from build123d import *

# Parameters (mm, degrees)
F1_DEPTH = 1.5
F2_DEPTH = 5
F3_ANGLE = 120
F4_ANGLE = 120
F6_DEPTH = 3


with BuildPart() as f1:
    # F0 (on Top) → F1 (new body)
    with BuildSketch(Plane.XY):
        Polygon((4.7835907286, 2.7618073949), (16.4544826719, 9.5), (9.3638996784, 13.59375), (8.2350135643, 12.5134618943), (6.7194691076, 13.3884618943), (7.0905829935, 14.90625), (0, 19), (0, 5.5236147897), (1.5310889132, 4.6396401935), (1.5310889132, 14.6519237886), (11.9233937587, 8.6519237886), (3.2525018154, 3.6457819911), align=None)
        Polygon((0, 0), (4.7835907286, 2.7618073949), (3.2525018154, 3.6457819911), (1.5310889132, 2.6519237886), (1.5310889132, 4.6396401935), (0, 5.5236147897), align=None)
        Polygon((-4.7835907286, 2.7618073949), (0, 0), (0, 5.5236147897), (-1.5310889132, 4.6396401935), (-1.5310889132, 2.6519237886), (-3.2525018154, 3.6457819911), align=None)
        Polygon((-1.5310889132, 4.6396401935), (0, 5.5236147897), (0, 19), (-6.7116968793, 15.125), (-7.0364564057, 14.9375), (-5.8534437039, 13.8884618943), (-9.101038968, 12.0134618943), (-9.4180262662, 13.5625), (-9.7427857926, 13.375), (-16.4544826719, 9.5), (-4.7835907286, 2.7618073949), (-3.2525018154, 3.6457819911), (-11.9233937587, 8.6519237886), (-1.5310889132, 14.6519237886), align=None)
    extrude(amount=F1_DEPTH)

    # F0 (on Top) → F2 (join)
    with BuildSketch(Plane.XY):
        Polygon((8.2350135643, 12.5134618943), (9.3638996784, 13.59375), (9.0888552775, 13.7525469589), (8.1894266762, 12.8918383296), (7.0699461568, 13.5381707088), (7.3656273944, 14.7474530411), (7.0905829935, 14.90625), (6.7194691076, 13.3884618943), align=None)
        Polygon((8.1894266762, 12.8918383296), (9.0888552775, 13.7525469589), (7.3656273944, 14.7474530411), (7.0699461568, 13.5381707088), align=None)
        Polygon((7.3656273944, 14.7474530411), (9.0888552775, 13.7525469589), (9.9882838789, 14.6132555882), (7.6613086319, 15.9567353735), align=None)
        Polygon((9.0888552775, 13.7525469589), (9.3638996784, 13.59375), (10.4927857926, 14.6740381057), (7.4616968793, 16.4240381057), (7.0905829935, 14.90625), (7.3656273944, 14.7474530411), (7.6613086319, 15.9567353735), (9.9882838789, 14.6132555882), align=None)
    extrude(amount=F2_DEPTH)


with BuildPart() as f3_1:
    # F3: copy of F1
    add(f1.part.rotate(Axis((0, 0, 0.75), (0, 0, -1)), F3_ANGLE))


with BuildPart() as f4_1:
    # F4: copy of F3_1
    add(f3_1.part.rotate(Axis((0, 0, 0.75), (0, 0, -1)), F4_ANGLE))


with BuildPart() as f1_1:
    add(f1.part)

    add(f3_1.part)  # F6 merges F3_1

    add(f4_1.part)  # F6 merges F4_1
    # F5 (on Top) → F6 (join)
    with BuildSketch(Plane.XY):
        Polygon((0.0358819761, -3.9998390572), (3.4819032227, -1.9688448258), (3.4460212466, 2.0309942315), (-0.0358819761, 3.9998390572), (-3.4819032227, 1.9688448258), (-3.4460212466, -2.0309942315), align=None)
    extrude(amount=F6_DEPTH)


solid = f1_1.part
Work out the finished part from the listing and answer in its coordinate system (mm). A direction names the side the tool comes from. Round coordinates to 2 decimals unless told otherwise and drop trailing zeros. Write each loop counter-clockwise with the first axis right and the second up, starting at its lowest first coordinate (ties: lowest second). Pieces come first, ordered by that corner, then holes. Notation, with made-up numbers: (-12, 66.25) - (5, 66.25) arc R25 ccw to (5, 102.25) - close; hole circle Ø1 at (46.25, 58). An arc over 180 degrees is marked (long way). Answer in a Markdown table with one row per item. Add a question column.
1. Given pin 1 (2 mm diameter, centred on x = 7, z = 2, fed in from +Y); pin 2 (1.2 mm diameter, centred on y = -12, z = 0.5, fed in from -X); pin 3 (1.6 mm diameter, centred on y = 7.5, z = 0.5, fed in from -X), each flat-ended and moving along its own axis, determine where each tip first touches the part or whether it passes through.
2. For faces 1 (the flat face through (15.69, 1.63, 0.74)), 2 (the flat face through (0, 0, 3)), 3 (the flat face through (-1.73, -3, 2.15)), determine the directions among +Z, -Z, +X, -X, +Y, -Y from which every point of the face is accessible in a straight line to the end or side of a thin tool.
3. The mould has two halves that part along Y. Classify faces 4 (the flat face through (15.715, -1.621, 0.74)), 5 (the flat face through (8.998, 15.537, 2.465)), 6 (the flat face through (-17, 0, 5)): +Y half, -Y half, draft (parallel to the pull), parting line (faces both ways), or undercut.
4. A cutting plane is placed at A-A, the plane z = 4.1. Count the separate pieces of the cut face and the enclosed holes in it, and give its area (3 significant figures).
5. A cutting plane is placed at B-B, the plane x = 4. Determine the outline of the cut face in (y, z).
6. Find the intervals of material crossed by line 1 along X through (y, z) = (0, 0.85); line 2 along Y through (x, z) = (-2.5, 0.35); line 3 along X through (y, z) = (-5, 1.05), in increasing order. Write a range as from..to.
7. A cutting plane is placed at D-D, the plane x = 14. Determine the outline of the cut face in (y, z).
Worked out:
| question | item | result |
|---|---|---|
| 1 | pin 1 | y = 16.42 |
| 1 | pin 2 | x = -13.16 |
| 1 | pin 3 | x = -16.45 |
| 2 | face 1 | +Z, -Z |
| 2 | face 2 | +Z, +X, +Y, -Y |
| 2 | face 3 | +Z |
| 3 | face 4 | undercut |
| 3 | face 5 | +Y half |
| 3 | face 6 | draft |
| 4 | separate pieces | 3 |
| 4 | enclosed holes | 0 |
| 4 | area | 23.6 mm^2 |
| 5 | outline | (-16.69, 0) - (-13.23, 0) - (-13.23, 1.5) - (-16.69, 1.5) - close; (-4.08, 0) - (-0.54, 0) - (-0.54, 1.5) - (-4.08, 1.5) - close; (0.54, 0) - (4.08, 0) - (4.08, 1.5) - (0.54, 1.5) - close; (13.23, 0) - (16.69, 0) - (16.69, 1.5) - (13.23, 1.5) - close |
| 6 | line 1 | -17.95..-13.45, -3.46..3.46, 13.45..14.95 |
| 6 | line 2 | -17.56..-14.09, -3.21..3.21, 14.09..17.56 |
| 6 | line 3 | -16.45..-13.45, -11.72..-5.6, -1.53..1.53, 5.6..11.72, 13.45..16.45 |
| 7 | outline | (-10.92, 0) - (10.92, 0) - (10.92, 1.5) - (-10.92, 1.5) - close |
